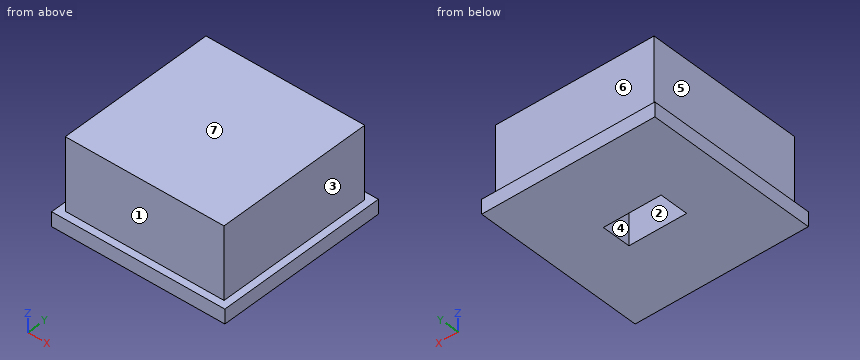
from build123d import *

# Parameters (mm, degrees)
F1_W     = 11
F1_H     = 11
F2_DEPTH = 6
F0_W     = 12
F0_H     = 12
F3_DEPTH = 1
F4_W     = 4
F4_H     = 2
F5_DEPTH = 4


with BuildPart() as f2:
    # F1 (on face) → F2 (new body)
    with BuildSketch(Plane.XY):
        Rectangle(F1_W, F1_H)
    extrude(amount=F2_DEPTH)

    # F0 (on Top) → F3 (join)
    with BuildSketch(Plane.XY):
        Rectangle(F0_W, F0_H)
    extrude(amount=F3_DEPTH)

    # F4 (on face) → F5 (cut)
    with BuildSketch(Plane(origin=(0, 0, 0), x_dir=(1, 0, 0), z_dir=(0, 0, -1))):
        Rectangle(F4_W, F4_H)
    extrude(amount=-F5_DEPTH, mode=Mode.SUBTRACT)


solid = f2.part
The listing builds one solid part. Answer for the finished solid, in the listing's coordinates (mm). Face numbers are marked on the shaded views. A direction names the side the tool comes from. Round coordinates to 2 decimals unless told otherwise and drop trailing zeros. Loops run counter-clockwise (first coordinate to the right, second up) from the corner with the lowest first, then second, coordinate; pieces in that order, holes last. Notation, with made-up numbers: M 14.25,59 L 32.25,59 A33 cw 32.25,98 Z; hole C 62,-25 d4. An arc over 180 degrees is marked long. Return JSON: item names as keys, results as strings.
Q1. Each of these flat-tipped pins is pushed along its axis until it touches: pin 1 Ø1.5 at (y, z) = (2, 3.5) entering from -X; pin 2 Ø1 at (x, y) = (0, 0) entering from -Z; pin 3 Ø0.6 at (y, z) = (0, 3) entering from +X. Where does it stop, or does it pass through?
Results list:
{"pin 1": "stops at x = -5.5", "pin 2": "stops at z = 4", "pin 3": "stops at x = 5.5"}
Q2. Find the intervals of material crossed by line 1 along Y through (x, z) = (-1, 3.05); line 2 along X through (y, z) = (-0.5, 0.8); line 3 along Y through (x, z) = (-1, 0.7), in increasing order. Write a range as from..to.
Results list:
{"line 1": "y = -5.5..-1, 1..5.5", "line 2": "x = -6..-2, 2..6", "line 3": "y = -6..-1, 1..6"}
Q3. Find section D-D, the plane z = 1.7. Determine the outline of the cut face in (x, y), plus the area to 3 significant figures.
Results list:
{"outline": "M -5.5,-5.5 L 5.5,-5.5 L 5.5,5.5 L -5.5,5.5 Z; hole M -2,-1 L 2,-1 L 2,1 L -2,1 Z", "area": "113 mm2"}
Q4. Find section B-B, the plane x = -3.25. Determine the outline of the cut face in (y, z), plus the area to 3 significant figures.
Results list:
{"outline": "M -6,0 L 6,0 L 6,1 L 5.5,1 L 5.5,6 L -5.5,6 L -5.5,1 L -6,1 Z", "area": "67.0 mm2"}
Q5. Find section C-C, the plane y = -0.5. Determine the outline of the cut face in (x, z), plus the area to 3 significant figures.
Results list:
{"outline": "M -6,0 L -2,0 L -2,4 L 2,4 L 2,0 L 6,0 L 6,1 L 5.5,1 L 5.5,6 L -5.5,6 L -5.5,1 L -6,1 Z", "area": "51.0 mm2"}
Q6. Find section A-A, the plane z = 0.55. Determine the outline of the cut face in (x, y), plus the area to 3 significant figures.
Results list:
{"outline": "M -6,-6 L 6,-6 L 6,6 L -6,6 Z; hole M -2,-1 L 2,-1 L 2,1 L -2,1 Z", "area": "136 mm2"}
Q7. Which of the six approach directions +Z, -Z, +X, -X, +Y, -Y give full straight-line access (tool end or side, diameter ignored) to the marked faces 5, 6 and 7?
Results list:
{"face 5": "+Z, -X, +Y, -Y", "face 6": "+Z, +X, -X, +Y", "face 7": "+Z, +X, -X, +Y, -Y"}
Q8. The mould has two halves that part along Y. Classify the marked faces 1, 2, 3 and 4: released by +Y, released by -Y, zero draft, split by the parting line, or undercut.
Results list:
{"face 1": "released by -Y", "face 2": "undercut", "face 3": "zero draft", "face 4": "undercut"}
